```python
from build123d import *

# Parameters (mm, degrees)
F0_R      = 2.55
F1_DEPTH  = 5
F2_DEPTH  = 25
F3_R      = 2.5
F5_DEPTH  = 3
F6_R      = 0.75
F8_D      = 5
F8_DEPTH  = 6
F10_D     = 5
F10_DEPTH = 6


with BuildPart() as f1:
    # F0 (on Top) → F1 (new body)
    with BuildSketch(Plane.XY):
        Polygon((-58, -25), (-83, -25), (-83, -30), (-64.919747, -30), (-30, -64.919747), (-30, -85), (-25, -85), (-25, -55), (-32.5, -55), (-58, -29.5), align=None)
        Polygon((0, 0), (-83, 0), (-83, -5), (-5, -5), (-5, -85), (0, -85), align=None)
        Polygon((-5, -5), (-83, -5), (-83, -25), (-58, -25), (-58, -29.5), (-32.5, -55), (-25, -55), (-25, -85), (-5, -85), align=None)
        with Locations((-40, -37)):
            Circle(F0_R, mode=Mode.SUBTRACT)
    extrude(amount=-F1_DEPTH)

    # F0 (on Top) → F2 (join)
    with BuildSketch(Plane.XY):
        Polygon((-58, -25), (-83, -25), (-83, -30), (-64.919747, -30), (-30, -64.919747), (-30, -85), (-25, -85), (-25, -55), (-32.5, -55), (-58, -29.5), align=None)
        Polygon((0, 0), (-83, 0), (-83, -5), (-5, -5), (-5, -85), (0, -85), align=None)
    extrude(amount=-F2_DEPTH)

    # F3
    f3_edges = [f1.edges().sort_by_distance(p)[0] for p in [
        (-73.959874, -30, 0),
        (-47.459874, -47.459874, 0),
        (-30, -74.959874, 0),
        (0, -42.5, 0),
        (-41.5, 0, 0),
        (0, 0, -12.5),
    ]]
    fillet(f3_edges, radius=F3_R)

    # F4 (on face) → F5 (cut)
    with BuildSketch(Plane.YZ.offset(-25)):
        Polygon((-55, -25), (-55, -5), (-69, -25), align=None)
    extrude(amount=-F5_DEPTH, mode=Mode.SUBTRACT)

    # F6
    f6_edges = [f1.edges().sort_by_distance(p)[0] for p in [
        (-58, -25, -15),
        (-28, -55, -15),
        (-25, -62, -15),
        (-5, -5, -15),
    ]]
    fillet(f6_edges, radius=F6_R)

    # F8
    with Locations(Plane(origin=(-30, 0, 0), x_dir=(0, -1, 0), z_dir=(-1, 0, 0))):
        with Locations((75, -15)):
            Hole(F8_D / 2, depth=F8_DEPTH)

    # F10
    with Locations(Plane.XZ.offset(30)):
        with Locations((-73.959874, -15)):
            Hole(F10_D / 2, depth=F10_DEPTH)


solid = f1.part
```
Here's how the part is built. I have some questions about the finished solid (model axes, mm). A direction names the side the tool comes from. Coordinates: 2 decimals unless noted, no trailing zeros. Order: outer loops, then holes, each group sorted by start corner. A loop starts at its lowest first (then second) coordinate and runs counter-clockwise, first axis right, second up.
1) We'd pull the mould along Y, two halves only. Please class faces 5 (the face through (-58, -28, -15)), 6 (the face through (-48, -46, -25)), 7 (the face through (-31, -55, -15)), 8 (the face through (-74, -30, -11)): +Y half, -Y half, draft (parallel to the pull), parting line (faces both ways), or undercut.
2) Which directions (+Z, -Z, +X, -X, +Y, -Y) give clear straight access to the entire face, cutting with the end or side of a thin tool? Please do faces 1 (the face through (-25, -74, -10)), 2 (the face through (-27.5, -77, -16.5)), 3 (the face through (-73.308, -29.287, -0.752)), 4 (the face through (-36, -36, -5)).
3) Imagine slicing it at C-C on y = -19. List the corners of the cut face in (x, z) for me.
4) I need wall thicknesses on line 1 (Y direction, x = -65.5, z = -9.5); line 2 (Z direction, x = -26.55, y = -75). Which ranges of each line are inside material? Lowest first, please.
5) Imagine slicing it at D-D on z = -15. State how many separate pieces and enclosed holes the cut face has, and give its area (3 significant figures).
6) Will these pins go through, and if not, where does the flat tip stop? pin 1 (8 mm diameter, centred on y = -72.5, z = -16, fed in from -X); pin 2 (4 mm diameter, centred on x = -29, y = -40, fed in from -Z); pin 3 (23.5 mm diameter, centred on x = -38, y = -38.5, fed in from -Z); pin 4 (8 mm diameter, centred on y = -50.5, z = -12.5, fed in from -X).
7) Imagine slicing it at B-B on x = -9. List the corners of the cut face in (y, z) for me, and give its area (3 significant figures).
8) Imagine slicing it at A-A on y = -75. List the corners of the cut face in (x, z) for me.
Response values:
1. face 5: undercut
1. face 6: draft
1. face 7: undercut
1. face 8: -Y half
2. face 1: -Z, -Y
2. face 2: -X
2. face 3: +Z, -X, -Y
2. face 4: -Z
3. outline: (-83, -5) - (-5, -5) - (-5, -25) - (0, -25) - (0, -2.5) arc R2.5 ccw to (-2.5, 0) - (-83, 0) - close
4. line 1: y = -30 to -25, -5 to 0
4. line 2: z = -25 to -17.5, -12.5 to 0
5. separate pieces: 4
5. enclosed holes: 0
5. area: 1,250 mm2
6. pin 1: stops at x = -30
6. pin 2: stops at z = -5
6. pin 3: stops at z = -25
6. pin 4: stops at x = -48.42
7. outline: (-85, -5) - (-5, -5) - (-5, -25) - (0, -25) - (0, -2.5) arc R2.5 ccw to (-2.5, 0) - (-85, 0) - close
7. area: 524 mm2
8. outline: (-30, -25) - (-25, -25) - (-25, -17.5) - (-30, -17.5) - close; (-30, -12.5) - (-25, -12.5) - (-25, -5) - (-5, -5) - (-5, -25) - (0, -25) - (0, -2.5) arc R2.5 ccw to (-2.5, 0) - (-27.5, 0) arc R2.5 ccw to (-30, -2.5) - close
